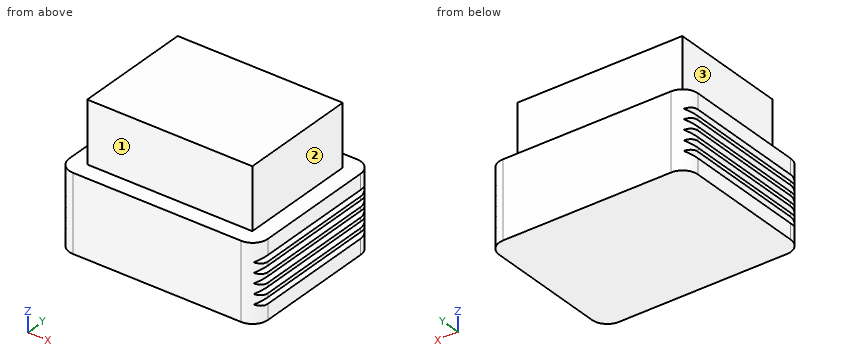
from build123d import *

# Parameters (mm, degrees)
F0_W     = 26
F0_H     = 20
F0_W_2   = 21.6
F0_H_2   = 15.6
F1_DEPTH = 10
F2_DEPTH = 18
F3_R     = 2
F5_DEPTH = 20


with BuildPart() as f1:
    # F0 (on Top) → F1 (new body)
    with BuildSketch(Plane.XY):
        with Locations((13, 10)):
            Rectangle(F0_W, F0_H)
        with Locations((13, 10)):
            Rectangle(F0_W_2, F0_H_2, mode=Mode.SUBTRACT)
    extrude(amount=F1_DEPTH)

    # F0 (on Top) → F2 (join)
    with BuildSketch(Plane.XY):
        with Locations((13, 10)):
            Rectangle(F0_W_2, F0_H_2)
    extrude(amount=F2_DEPTH)

    # F3
    f3_edges = [f1.edges().sort_by_distance(p)[0] for p in [
        (26, 0, 5),
        (26, 20, 5),
        (0, 20, 5),
        (0, 0, 5),
    ]]
    fillet(f3_edges, radius=F3_R)

    # F4 (on face) → F5 (cut, through all)
    with BuildSketch(Plane.XZ):
        Polygon((26, 1.9958548116), (26, 2.8041451884), (25.3, 2.4), align=None)
        Polygon((26, 3.2958548116), (26, 4.1041451884), (25.3, 3.7), align=None)
        Polygon((26.35, 3.0062177826), (26, 2.8041451884), (26, 1.9958548116), (26.35, 1.7937822174), align=None)
        Polygon((26.35, 4.3062177826), (26, 4.1041451884), (26, 3.2958548116), (26.35, 3.0937822174), align=None)
        Polygon((26.35, 5.6062177826), (26, 5.4041451884), (26, 4.5958548116), (26.35, 4.3937822174), align=None)
        Polygon((26, 4.5958548116), (26, 5.4041451884), (25.3, 5), align=None)
        Polygon((26.35, 6.9062177826), (26, 6.7041451884), (26, 5.8958548116), (26.35, 5.6937822174), align=None)
        Polygon((26, 5.8958548116), (26, 6.7041451884), (25.3, 6.3), align=None)
        Polygon((26, 7.1958548116), (26, 8.0041451884), (25.3, 7.6), align=None)
        Polygon((26.35, 8.2062177826), (26, 8.0041451884), (26, 7.1958548116), (26.35, 6.9937822174), align=None)
        Polygon((0, 8.0041451884), (0, 7.1958548116), (0.7, 7.6), align=None)
        Polygon((0, 6.7041451884), (0, 5.8958548116), (0.7, 6.3), align=None)
        Polygon((0, 5.4041451884), (0, 4.5958548116), (0.7, 5), align=None)
        Polygon((0, 4.1041451884), (0, 3.2958548116), (0.7, 3.7), align=None)
        Polygon((-0.35, 6.9937822174), (0, 7.1958548116), (0, 8.0041451884), (-0.35, 8.2062177826), align=None)
        Polygon((-0.35, 5.6937822174), (0, 5.8958548116), (0, 6.7041451884), (-0.35, 6.9062177826), align=None)
        Polygon((0, 2.8041451884), (0, 1.9958548116), (0.7, 2.4), align=None)
        Polygon((-0.35, 4.3937822174), (0, 4.5958548116), (0, 5.4041451884), (-0.35, 5.6062177826), align=None)
        Polygon((-0.35, 3.0937822174), (0, 3.2958548116), (0, 4.1041451884), (-0.35, 4.3062177826), align=None)
        Polygon((-0.35, 1.7937822174), (0, 1.9958548116), (0, 2.8041451884), (-0.35, 3.0062177826), align=None)
    extrude(amount=-F5_DEPTH, mode=Mode.SUBTRACT)


solid = f1.part
The model under review builds one solid part; all positions refer to its coordinate system, in mm. Face numbers are marked on the shaded views. A direction names the side the tool comes from. Give positions to 0.01 mm unless a question says otherwise; leave off trailing zeros. Order: outer loops, then holes, each group sorted by start corner. A loop starts at its lowest first (then second) coordinate and runs counter-clockwise, first axis right, second up. Notation, with made-up numbers: M 2.25,62 L 17.25,62 A24 cw 17.25,84 Z; hole C 77,-12 d11. An arc over 180 degrees is marked long. Answer in a Markdown table with one row per item. Add a question column.
1. Add section B-B on z = 12.5. State the section outline as (x, y) points, plus the area to 3 significant figures.
2. Add section A-A on x = 10.5. State the section outline as (y, z) points, plus the area to 3 significant figures.
3. To check wall thickness, follow line 1 along X through (y, z) = (6.5, 16); line 2 along Y through (x, z) = (13.75, 11.5); line 3 along Z through (x, y) = (25, 6.75). State the ranges of each line that lie inside material, in increasing order.
4. For pin 1 Ø6.5 at (x, z) = (14, 14) entering from -Y; pin 2 Ø2.5 at (x, z) = (12, 14.5) entering from +Y; pin 3 Ø10 at (y, z) = (7.5, 15.5) entering from -X, all flat-tipped, find the tip position at first contact; note any pin that passes through.
5. Machinability: for the marked faces 1, 2 and 3, which of the approach directions +Z, -Z, +X, -X, +Y, -Y give a long, thin tool a straight path to every point of the face, cutting with its end or side? Answer none if there is none.
The answers:
| question | item | result |
|---|---|---|
| 1 | outline | M 2.2,2.2 L 23.8,2.2 L 23.8,17.8 L 2.2,17.8 Z |
| 1 | area | 337 mm2 |
| 2 | outline | M 0,0 L 20,0 L 20,10 L 17.8,10 L 17.8,18 L 2.2,18 L 2.2,10 L 0,10 Z |
| 2 | area | 325 mm2 |
| 3 | line 1 | 2.2 to 23.8 |
| 3 | line 2 | 2.2 to 17.8 |
| 3 | line 3 | 0 to 10 |
| 4 | pin 1 | y = 2.2 |
| 4 | pin 2 | y = 17.8 |
| 4 | pin 3 | x = 2.2 |
| 5 | face 1 | +Z, +X, -X, -Y |
| 5 | face 2 | +Z, +X, +Y, -Y |
| 5 | face 3 | +Z, -X, +Y, -Y |
